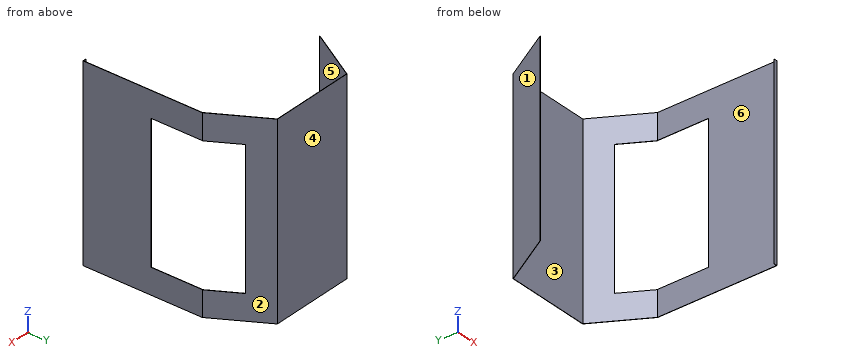
Autodesk Inventor part; units mm, degrees
ref_plane "YZ Plane" through (0, 0, 0) normal (1, 0, 0) x (0, 1, 0)
ref_plane "XZ Plane" through (0, 0, 0) normal (0, 1, 0) x (-1, 0, 0)
ref_plane "XY Plane" through (0, 0, 0) normal (0, 0, 1) x (1, 0, 0)
sketch "Sketch1" plane through (0, 0, 0) normal (0, 0, 1) x (1, 0, 0)
  line L0 (0, 0) -> (20, 0)
  line L1 (20, 0) -> (20, 700)
  line L2 (20, 700) -> (-153, 999.6448)
  line L3 (-153, 999.6448) -> (-653, 999.6448)
  line L4 (-653, 999.6448) -> (-826, 700)
  line L5 (-824.1525, 700) -> (-652.0762, 998.0448)
  line L6 (-652.0762, 998.0448) -> (-153.9238, 998.0448)
  line L7 (-153.9238, 998.0448) -> (18.4, 699.5713)
  line L8 (18.4, 699.5713) -> (18.4, 1.6)
  line L9 (18.4, 1.6) -> (0, 1.6)
  line L10 (-826, 700) -> (-824.1525, 700)
  line L11 (0, 1.6) -> (0, 0)
  dimension "d0" = 20
  dimension "d1" = 700
  dimension "d2" = 90
  dimension "d3" = 346
  dimension "d4" = 150
  dimension "d5" = 500
  dimension "d6" = 346
  dimension "d7" = 120
  dimension "d8" = 1.6
extrude "main" add sketch "Sketch1" along normal blind 1100
sketch "Sketch2" plane through (20, 0, 0) normal (1, 0, 0) x (0, 0, -1)
  point P0 (0, 0)
sketch "Sketch3" plane through (20, 0, 0) normal (1, 0, 0) x (0, 0, -1)
  line L0 (-1100, 0) -> (-1100, 700)
  line L1 (-950, 400) -> (-150, 400)
  line L2 (-150, 400) -> (-150, 700)
  line L3 (-150, 700) -> (-950, 700)
  line L4 (-950, 700) -> (-950, 400)
  line L5 (-950, 700) -> (-150, 700)
  point P0 (0, 0)
  dimension "d13" = 800
  dimension "d14" = 300
sketch "Sketch4" plane through (-153, 999.6448, 1100) normal (0.866, 0.5, 0) x (0, 0, -1)
  line L0 (1100, -346) -> (0, -346)
  line L1 (151.2631, -346) -> (951.2631, -346)
  line L2 (951.2631, -346) -> (951.2631, -146)
  line L3 (951.2631, -146) -> (151.2631, -146)
  line L4 (151.2631, -146) -> (151.2631, -346)
  point P0 (1100, -942.2178)
  dimension "d16" = 800
  dimension "d17" = 200
extrude "Extrusion2" cut sketch "Sketch4" against normal blind 1.6
extrude "Extrusion3" cut sketch "Sketch3" against normal blind 1.6
properties part number "Cover 1"
Input: part model. Units: mm. Frame: model coordinates. Face numbers are marked on the shaded views. A direction names the side the tool comes from. Give positions to 0.01 mm unless a question says otherwise; leave off trailing zeros. Write each loop counter-clockwise with the first axis right and the second up, starting at its lowest first coordinate (ties: lowest second). Pieces come first, ordered by that corner, then holes.
Q1. First-contact query: P1, Ø0.6, axis at x = -825.5, z = 758.5, coming from the -Y side; P2, Ø6, axis at y = 175.5, z = 976, coming from the -X side; P3, Ø5.5, axis at x = 6.5, z = 529, coming from the +Y side. Flat tips, straight axial feed; report the tip coordinate or a pass-through.
Q2. Set-up query: the marked faces 4, 5 and 6. Return all of +Z, -Z, +X, -X, +Y, -Y with unobstructed straight access to the full face (end or side cutting, diameter ignored); none if empty.
Q3. Section B-B, the plane z = 884.5. Output: boundary loops of the cut face in (x, y), plus the area to 3 significant figures.
Q4. Section D-D, the plane z = 92.5. Output: boundary loops of the cut face in (x, y), plus the area to 3 significant figures.
Q5. Pull-direction query (X, two-part tool) for the marked faces 1, 2 and 3; classes: pulls with the +X half, pulls with the -X half, needs draft (parallel to the pull), parting line crosses it, or undercut.
Q6. Material intervals for probe 1 along Y at (x, z) = (-354.5, 478); probe 2 along X at (y, z) = (263, 708.5); probe 3 along X at (y, z) = (853, 66.5), sorted ascending.
Q7. Section C-C, the plane y = 858. Output: boundary loops of the cut face in (x, z), plus the area to 3 significant figures.
Q8. Section A-A, the plane y = 645.5. Output: boundary loops of the cut face in (x, z), plus the area to 3 significant figures.
Filled in:
1. P1: stops at y = 700
1. P2: stops at x = 18.4
1. P3: stops at y = 1.6
2. face 4: +Z, -Z, +X, -X, +Y
2. face 5: +Z, -Z, -Y
2. face 6: +Z, -Z, -X
3. outline: (-826, 700) - (-824.15, 700) - (-652.08, 998.04) - (-153.92, 998.04) - (-81.39, 872.41) - (-80, 873.21) - (-153, 999.64) - (-653, 999.64) - close; (0, 0) - (20, 0) - (20, 400) - (18.4, 400) - (18.4, 1.6) - (0, 1.6) - close
3. area: 2,250 mm2
4. outline: (-826, 700) - (-824.15, 700) - (-652.08, 998.04) - (-153.92, 998.04) - (18.4, 699.57) - (18.4, 1.6) - (0, 1.6) - (0, 0) - (20, 0) - (20, 700) - (-153, 999.64) - (-653, 999.64) - close
4. area: 3,050 mm2
5. face 1: pulls with the -X half
5. face 2: pulls with the +X half
5. face 3: undercut
6. probe 1: y = 998.04 to 999.64
6. probe 2: x = 18.4 to 20
6. probe 3: x = -737.67 to -735.82, -70.18 to -68.33
7. outline: (-734.78, 0) - (-732.93, 0) - (-732.93, 1100) - (-734.78, 1100) - close; (-73.07, 0) - (-71.22, 0) - (-71.22, 148.74) - (-73.07, 148.74) - close; (-73.07, 948.74) - (-71.22, 948.74) - (-71.22, 1100) - (-73.07, 1100) - close
7. area: 2,590 mm2
8. outline: (18.4, 0) - (20, 0) - (20, 150) - (18.4, 150) - close; (18.4, 950) - (20, 950) - (20, 1100) - (18.4, 1100) - close
8. area: 480 mm2
